Geometry: final body of the model. Coordinates: model frame, mm. A direction names the side the tool comes from. Give positions to 0.01 mm unless a question says otherwise; leave off trailing zeros. Loops run counter-clockwise (first coordinate to the right, second up) from the corner with the lowest first, then second, coordinate; pieces in that order, holes last.
1. Section B-B, the plane x = -4.5. Output: boundary loops of the cut face in (y, z), then the cut area to 3 significant figures.
2. First-contact query: P1, Ø3, axis at y = -2.5, z = 3, coming from the -X side; P2, Ø7.5, axis at x = -6.5, z = 3.5, coming from the -Y side. Flat tips, straight axial feed; report the tip coordinate or a pass-through.
3. Draft query along Z for faces 1 (the face through (-5.716, -4.858, -14.635)), 2 (the face through (-5, -6, -11.5)), 3 (the face through (-8, -5, 20)), 4 (the face through (0, 0.3, 0.3)). Return one class per face: +Z half, -Z half, draft (parallel to the pull), parting line (faces both ways), or undercut.
4. Section C-C, the plane z = -15.75. Output: boundary loops of the cut face in (x, y).
5. Section A-A, the plane y = -3.25. Output: boundary loops of the cut face in (x, z), then the cut area to 3 significant figures.
6. Material intervals for line 1 along Z through (x, y) = (-4.5, -7.5); line 2 along Z through (x, y) = (-14, -9); line 3 along Z through (x, y) = (-10, -8.5), sorted ascending.
7. Access query for faces 5 (the face through (-5, -6, 11.5)), 6 (the face through (-8, -12.5, -16)), 7 (the face through (-10, -6, -16.5)). Directions: +Z, -Z, +X, -X, +Y, -Y. A direction counts if a zero-diameter tool reaches every point of the face in a straight line with its end or side. Return the directions, or none.
8. Section D-D, the plane y = 0.5. Output: boundary loops of the cut face in (x, z), then the cut area to 3 significant figures.
Autodesk Inventor part; units mm, degrees
ref_plane "YZ Plane" through (0, 0, 0) normal (1, 0, 0) x (0, 1, 0)
ref_plane "XZ Plane" through (0, 0, 0) normal (0, 1, 0) x (-1, 0, 0)
ref_plane "XY Plane" through (0, 0, 0) normal (0, 0, 1) x (1, 0, 0)
sketch "Эскиз1" plane through (0, 0, 0) normal (0, 1, 0) x (-1, 0, 0)
  line L0 (0, 0) -> (-10.5018, 0)
  line L1 (0, 0) -> (15, 0)
  line L2 (15, 0) -> (15, -20)
  line L3 (15, -20) -> (0, -20)
  line L4 (0, -20) -> (0, 0)
  line L5 (15, 0) -> (15, 20)
  line L6 (15, 20) -> (0, 20)
  line L7 (0, 20) -> (0, 0)
  dimension "d5" = 15
  dimension "d6" = 20
extrude "Выдавливание1" add sketch "Эскиз1" along normal blind 3
sketch "Эскиз3" plane through (0, 0, 0) normal (0, -1, 0) x (1, 0, 0)
  line L0 (-15, 20) -> (0, 20)
  line L1 (-9, 16.5) -> (-11.5, 16.5)
  line L2 (-11.5, 16.5) -> (-11.5, 11.5)
  line L3 (-9, 11.5) -> (-9, 16.5)
  line L4 (0, 0) -> (-5.7861, 0)
  line L5 (-9, -16.5) -> (-11.5, -16.5)
  line L6 (-11.5, -16.5) -> (-11.5, -11.5)
  line L7 (-9, -11.5) -> (-9, -16.5)
  line L8 (-9, -11.5) -> (0, -11.5)
  line L9 (0, 20) -> (0, -20)
  line L10 (0, -20) -> (-15, -20)
  line L11 (0, -20) -> (-15, -20)
  line L12 (-15, -20) -> (-15, -11.5)
  line L13 (-15, -20) -> (-15, 20)
  line L14 (-11.5, -11.5) -> (-15, -11.5)
  line L15 (0, -11.5) -> (0, -20)
  line L16 (-11.5, 16.5) -> (-11.5, 11.5)
  line L17 (-9, 11.5) -> (-9, 16.5)
  line L18 (-9, 16.5) -> (-11.5, 16.5)
  line L19 (-9, 11.5) -> (0, 11.5)
  line L20 (0, 20) -> (-15, 20)
  line L21 (0, 20) -> (-15, 20)
  line L22 (-15, 20) -> (-15, 11.5)
  line L23 (-11.5, 11.5) -> (-15, 11.5)
  line L24 (0, 11.5) -> (0, 20)
  point P0 (-15, 11.5)
extrude "Выдавливание2" add sketch "Эскиз3" along normal blind 12.5 contours L0 L9 L19 L3 L1 L2 L23 L13 | L14 L6 L5 L7 L8 L9 L10 L12
sketch "Эскиз4" plane through (0, -12.5, 0) normal (0, -1, 0) x (1, 0, 0)
  line L0 (-15, 20) -> (0, 20)
  line L1 (0, 20) -> (-4.5, 20)
  circle A0 centre (-4.5, 15.75) radius 1.65
  line L2 (0, 0) -> (-4.5, 0)
  circle A1 centre (-4.5, -15.75) radius 1.65
  dimension "d18" = 3.3
extrude "Выдавливание3" cut sketch "Эскиз4" against normal through all
sketch "Эскиз5" plane through (-11.5, 0, -11.5) normal (1, 0, 0) x (0, 0, -1)
  line L0 (0, -12.5) -> (8.5, -12.5)
  line L1 (4.25, -12.5) -> (4.25, -6)
  line L2 (0, -6) -> (3.191, -6)
  circle A0 centre (3.191, -6) radius 1.1
  line L3 (-11.5, 0) -> (-11.5, -8.8463)
  circle A1 centre (-26.191, -6) radius 1.1
  dimension "d20" = 3.191
  dimension "d21" = 2.2
properties part number "держалка_серво_бровь_нижняя"
Answers below:
1. outline: (-12.5, -20) - (3, -20) - (3, -17.4) - (-12.5, -17.4) - close; (-12.5, -14.1) - (3, -14.1) - (3, 14.1) - (-12.5, 14.1) - (-12.5, 11.5) - (0, 11.5) - (0, -11.5) - (-12.5, -11.5) - close; (-12.5, 17.4) - (3, 17.4) - (3, 20) - (-12.5, 20) - close
1. area: 230 mm2
2. P1: passes through
2. P2: stops at y = 0
3. face 1: undercut
3. face 2: undercut
3. face 3: +Z half
3. face 4: draft
4. outline: (-15, -12.5) - (-11.5, -12.5) - (-11.5, 0) - (-9, 0) - (-9, -12.5) - (-6.15, -12.5) - (-6.15, 3) - (-15, 3) - close; (-2.85, -12.5) - (0, -12.5) - (0, 3) - (-2.85, 3) - close
5. outline: (-15, -20) - (0, -20) - (0, -11.5) - (-9, -11.5) - (-9, -16.5) - (-11.5, -16.5) - (-11.5, -11.5) - (-15, -11.5) - close; (-15, 11.5) - (-11.5, 11.5) - (-11.5, 16.5) - (-9, 16.5) - (-9, 11.5) - (0, 11.5) - (0, 20) - (-15, 20) - close; hole circle Ø3.3 at (-4.5, -15.75); hole circle Ø3.3 at (-4.5, 15.75)
5. area: 213 mm2
6. line 1: z = -20 to -17.4, -14.1 to -11.5, 11.5 to 14.1, 17.4 to 20
6. line 2: z = -20 to -11.5, 11.5 to 20
6. line 3: z = -20 to -16.5, 16.5 to 20
7. face 5: +X, -X, -Y
7. face 6: +Z, -Z, +X, -X, -Y
7. face 7: -Y
8. outline: (-15, -20) - (0, -20) - (0, 20) - (-15, 20) - close; hole circle Ø3.3 at (-4.5, -15.75); hole circle Ø3.3 at (-4.5, 15.75)
8. area: 583 mm2
